from build123d import *

# Parameters (mm, degrees)
F0_W     = 80
F0_H     = 80
F1_DEPTH = 25
F2_R     = 5
F4_D     = 5
F5_T     = -2.5


with BuildPart() as f1:
    # F0 (on Top) → F1 (new body)
    with BuildSketch(Plane.XY):
        with Locations((12.7454949915, 13.8860409707)):
            Rectangle(F0_W, F0_H)
    extrude(amount=F1_DEPTH)

    # F2
    f2_edges = [f1.edges().sort_by_distance(p)[0] for p in [
        (52.745495, 13.886041, 25),
        (12.745495, -26.113959, 25),
        (-27.254505, 13.886041, 25),
        (12.745495, 53.886041, 25),
    ]]
    fillet(f2_edges, radius=F2_R)

    # F4 (through all)
    with Locations(Plane.XY.offset(25)):
        with Locations((12.1779767796, 12.7649977803)):
            Hole(F4_D / 2)

    # F5
    f5_openings = [f1.faces().sort_by_distance(p)[0] for p in [
        (-26.123134, 13.886041, 0),
    ]]
    offset(amount=F5_T, openings=f5_openings)


solid = f1.part
Source: CAD feature listing. Evaluate the final solid. Frame: model axes, mm. A direction names the side the tool comes from. Coordinates: 2 decimals unless noted, no trailing zeros. Order: outer loops, then holes, each group sorted by start corner. A loop starts at its lowest first (then second) coordinate and runs counter-clockwise, first axis right, second up.
Item 1: Cut plane A-A (z = 7). Return loops of the section in (x, y) (1 decimal).
Output values:
outline: (-27.3, -26.1) - (52.7, -26.1) - (52.7, 53.9) - (-27.3, 53.9) - close; circle Ø10 at (12.2, 12.8); hole (-24.8, -23.6) - (50.2, -23.6) - (50.2, 51.4) - (-24.8, 51.4) - close; hole circle Ø5 at (12.2, 12.8)
Item 2: Cut plane B-B (y = 28). Return loops of the section in (x, z), plus the area to 3 significant figures.
Output values:
outline: (-27.25, 0) - (-24.75, 0) - (-24.75, 20) arc R2.5 cw to (-22.25, 22.5) - (47.75, 22.5) arc R2.5 cw to (50.25, 20) - (50.25, 0) - (52.75, 0) - (52.75, 20) arc R5 ccw to (47.75, 25) - (-22.25, 25) arc R5 ccw to (-27.25, 20) - close
area: 304 mm2
Item 3: Pull-direction query (X, two-part tool) for faces 1 (the face through (-27.255, 13, 10)), 2 (the face through (4, 14, 22.5)), 3 (the face through (52.745, 13, 10)), 4 (the face through (12, -23.614, 10)); classes: pulls with the +X half, pulls with the -X half, needs draft (parallel to the pull), parting line crosses it, or undercut.
Output values:
face 1: pulls with the -X half
face 2: undercut
face 3: pulls with the +X half
face 4: undercut
Item 4: Material intervals for line 1 (Y direction, x = -5.5, z = 6); line 2 (X direction, y = 12.5, z = 2.5) (1 decimal); line 3 (X direction, y = 23.5, z = 6), sorted ascending.
Output values:
line 1: y = -26.11 to -23.61, 51.39 to 53.89
line 2: x = -27.3 to -24.8, 7.2 to 9.7, 14.7 to 17.2, 50.2 to 52.7
line 3: x = -27.25 to -24.75, 50.25 to 52.75
Item 5: First-contact query: P1, Ø1.5, axis at x = -5.5, y = -12.5, coming from the -Z side. Flat tip, straight axial feed; report the tip coordinate or a pass-through.
Output values:
P1: stops at z = 22.5
Item 6: Cut plane D-D (z = 23.5). Return loops of the section in (x, y) (3 decimals).
Output values:
outline: (-25.825, -24.685) - (51.316, -24.685) - (51.316, 52.457) - (-25.825, 52.457) - close; hole circle Ø5 at (12.178, 12.765)
Item 7: Set-up query: faces 5 (the face through (13.27, -22.9, 21.75)), 6 (the face through (13.305, -24.688, 23.496)). Return all of +Z, -Z, +X, -X, +Y, -Y with unobstructed straight access to the full face (end or side cutting, diameter ignored); none if empty.
Output values:
face 5: -Z
face 6: +Z, +X, -X, -Y
Item 8: Cut plane C-C (x = -3). Return loops of the section in (y, z), plus the area to 3 significant figures.
Output values:
outline: (-26.11, 0) - (-23.61, 0) - (-23.61, 20) arc R2.5 cw to (-21.11, 22.5) - (48.89, 22.5) arc R2.5 cw to (51.39, 20) - (51.39, 0) - (53.89, 0) - (53.89, 20) arc R5 ccw to (48.89, 25) - (-21.11, 25) arc R5 ccw to (-26.11, 20) - close
area: 304 mm2
